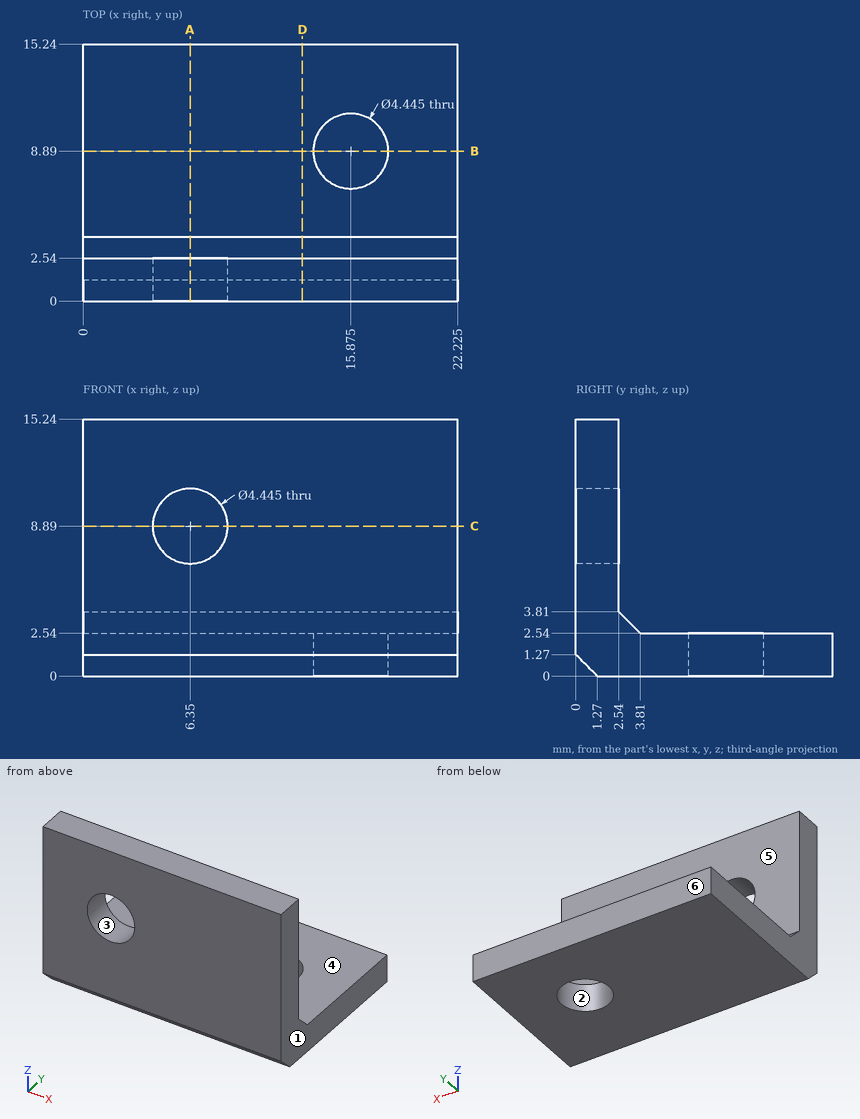
Source: three-view drawing plus pictorial views. Frame: mm from the lowest corner of the part. A direction names the side the tool comes from. Round coordinates to 2 decimals unless told otherwise and drop trailing zeros. Order: outer loops, then holes, each group sorted by start corner. A loop starts at its lowest first (then second) coordinate and runs counter-clockwise, first axis right, second up. Notation, with made-up numbers: (67, 64) - (74, 64) arc R17 cw to (74, 71) - close; hole circle Ø10 at (32.5, 71). An arc over 180 degrees is marked (long way). Write each question's results on one line, items separated by ' | '.
Item 1: Mould query, pull axis X, two halves, no side actions, for the marked faces 1, 2, 3 and 4. Classes: pulls with the +X half, pulls with the -X half, needs draft (parallel to the pull), parting line crosses it, or undercut.
Completed:
face 1: pulls with the +X half | face 2: undercut | face 3: undercut | face 4: needs draft
Item 2: Section D-D, the plane x = 13. Return the cut outline in (y, z).
Completed:
outline: (0, 1.27) - (1.27, 0) - (15.24, 0) - (15.24, 2.54) - (3.81, 2.54) - (2.54, 3.81) - (2.54, 15.24) - (0, 15.24) - close
Item 3: Section B-B, the plane y = 8.89. Return the cut outline in (x, z) (1 decimal), and give its area (3 significant figures).
Completed:
outline: (0, 0) - (13.7, 0) - (13.7, 2.5) - (0, 2.5) - close; (18.1, 0) - (22.2, 0) - (22.2, 2.5) - (18.1, 2.5) - close | area: 45.2 mm^2
Item 4: First-contact query: pin 1 Ø5.5 at (x, y) = (16.5, 9.5) entering from +Z. Flat tip, straight axial feed; report the tip coordinate or a pass-through.
Completed:
pin 1: z = 2.54
Item 5: Material intervals for line 1 along Y through (x, z) = (7.25, 4.25); line 2 along Z through (x, y) = (6.35, 1.7); line 3 along Y through (x, z) = (17.25, 2.5), sorted ascending. Write a range as [from, to].
Completed:
line 1: [0, 2.54] | line 2: [0, 6.67], [11.11, 15.24] | line 3: [0, 7.14], [10.64, 15.24]
Item 6: Section A-A, the plane x = 6.35. Return the cut outline in (y, z), and give its area (3 significant figures).
Completed:
outline: (0, 1.27) - (1.27, 0) - (15.24, 0) - (15.24, 2.54) - (3.81, 2.54) - (2.54, 3.81) - (2.54, 6.67) - (0, 6.67) - close; (0, 11.11) - (2.54, 11.11) - (2.54, 15.24) - (0, 15.24) - close | area: 59.7 mm^2
Item 7: Reachability of the marked faces 5 and 6 from +Z, -Z, +X, -X, +Y, -Y: full face, straight path, thin tool, end or side. Return the list, or none.
Completed:
face 5: +Z, +X, -X, +Y | face 6: +Z, -Z, +X, -X, +Y
Item 8: Section C-C, the plane z = 8.89. Return the cut outline in (x, y) (1 decimal), and give its area (3 significant figures).
Completed:
outline: (0, 0) - (4.1, 0) - (4.1, 2.5) - (0, 2.5) - close; (8.6, 0) - (22.2, 0) - (22.2, 2.5) - (8.6, 2.5) - close | area: 45.2 mm^2
